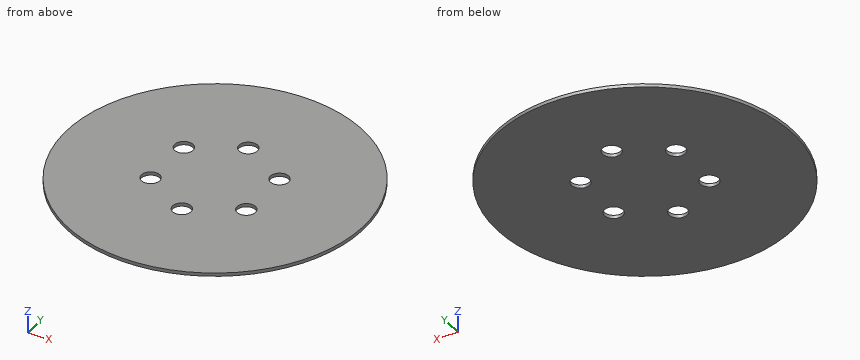
from build123d import *

# Parameters (mm, degrees)
SKETCH1_R           = 44.22
SKETCH1_R_2         = 2.75
BOSS_EXTRUDE1_DEPTH = 1


with BuildPart() as part:
    # Sketch1 → Boss-Extrude1 (new body)
    with BuildSketch(Plane.XY):
        with Locations((0, 1.049337112)):
            Circle(SKETCH1_R)
        with Locations((0, 17.619337112)):
            Circle(SKETCH1_R_2, mode=Mode.SUBTRACT)
        with Locations((14.350040941, 9.334337112)):
            Circle(SKETCH1_R_2, mode=Mode.SUBTRACT)
        with Locations((14.350040941, -7.235662888)):
            Circle(SKETCH1_R_2, mode=Mode.SUBTRACT)
        with Locations((0, -15.520662888)):
            Circle(SKETCH1_R_2, mode=Mode.SUBTRACT)
        with Locations((-14.350040941, -7.235662888)):
            Circle(SKETCH1_R_2, mode=Mode.SUBTRACT)
        with Locations((-14.350040941, 9.334337112)):
            Circle(SKETCH1_R_2, mode=Mode.SUBTRACT)
    extrude(amount=BOSS_EXTRUDE1_DEPTH)


solid = part.part
Geometry check sheet. Reference: the model listing, model coordinates, mm. Give positions to 0.01 mm unless a question says otherwise; leave off trailing zeros. Order: outer loops, then holes, each group sorted by start corner. A loop starts at its lowest first (then second) coordinate and runs counter-clockwise, first axis right, second up.
1. Sectioned sample at C-C (y = 31). Record the boundary of the cut face in (x, z).
Completed:
outline: (-32.53, 0) - (32.53, 0) - (32.53, 1) - (-32.53, 1) - close
2. Sectioned sample at D-D (x = 24.5). Record the boundary of the cut face in (y, z).
Completed:
outline: (-35.76, 0) - (37.86, 0) - (37.86, 1) - (-35.76, 1) - close
3. Sectioned sample at B-B (z = 0.7). Record the boundary of the cut face in (x, y).
Completed:
outline: circle Ø88.44 at (0, 1.05); hole circle Ø5.5 at (-14.35, -7.24); hole circle Ø5.5 at (-14.35, 9.33); hole circle Ø5.5 at (0, -15.52); hole circle Ø5.5 at (0, 17.62); hole circle Ø5.5 at (14.35, -7.24); hole circle Ø5.5 at (14.35, 9.33)
4. Sectioned sample at A-A (x = 0). Record the boundary of the cut face in (y, z).
Completed:
outline: (-43.17, 0) - (-18.27, 0) - (-18.27, 1) - (-43.17, 1) - close; (-12.77, 0) - (14.87, 0) - (14.87, 1) - (-12.77, 1) - close; (20.37, 0) - (45.27, 0) - (45.27, 1) - (20.37, 1) - close
5. Scan lines: line 1 (Y direction, x = 0, z = 0.2); line 2 (X direction, y = 8, z = 0.1); line 3 (Y direction, x = -15, z = 0.2). Record each from-to range of solid material in increasing order.
Completed:
line 1: y = -43.17 to -18.27, -12.77 to 14.87, 20.37 to 45.27
line 2: x = -43.67 to -16.75, -11.95 to 11.95, 16.75 to 43.67
line 3: y = -40.55 to -9.91, -4.56 to 6.66, 12.01 to 42.65
